from build123d import *

# Parameters (mm, degrees)
BOSS_EXTRUDE1_DEPTH = 3
SKETCH2_W           = 3
SKETCH2_H           = 3
CUT_EXTRUDE1_DEPTH  = 3
SKETCH3_R           = 1.5
CUT_EXTRUDE2_DEPTH  = 3
SKETCH4_W           = 3
SKETCH4_H           = 6
SKETCH4_H_2         = 3
CUT_EXTRUDE3_DEPTH  = 10


with BuildPart() as part:
    # Sketch1 → Boss-Extrude1 (new body)
    with BuildSketch(Plane(origin=(0, 0, 0), x_dir=(0, 0, -1), z_dir=(1, 0, 0))):
        Polygon((8, 30), (12.5, 30), (12.5, -30), (8, -30), (8, -27), (2, -27), (2, -30), (-2, -30), (-2, -27), (-8, -27), (-8, -30), (-12.5, -30), (-12.5, 30), (-8, 30), (-8, 27), (-2, 27), (-2, 30), (2, 30), (2, 27), (8, 27), align=None)
    extrude(amount=BOSS_EXTRUDE1_DEPTH)

    # Sketch2 → Cut-Extrude1 (cut)
    with BuildSketch(Plane(origin=(3, 0, 0), x_dir=(0, 0, -1), z_dir=(1, 0, 0))):
        with Locations((-5, 22.5)):
            Rectangle(SKETCH2_W, SKETCH2_H)
        with Locations((5, 22.5)):
            Rectangle(SKETCH2_W, SKETCH2_H)
        with Locations((5, -22.5)):
            Rectangle(SKETCH2_W, SKETCH2_H)
        with Locations((-5, -22.5)):
            Rectangle(SKETCH2_W, SKETCH2_H)
    extrude(amount=-CUT_EXTRUDE1_DEPTH, mode=Mode.SUBTRACT)

    # Sketch3 → Cut-Extrude2 (cut)
    with BuildSketch(Plane(origin=(3, 0, 0), x_dir=(0, 0, -1), z_dir=(1, 0, 0))):
        Circle(SKETCH3_R)
        with Locations((10, 0)):
            Circle(SKETCH3_R)
    extrude(amount=-CUT_EXTRUDE2_DEPTH, mode=Mode.SUBTRACT)

    # Sketch4 → Cut-Extrude3 (cut)
    with BuildSketch(Plane(origin=(3, 0, 0), x_dir=(0, 0, -1), z_dir=(1, 0, 0))):
        with Locations((-11, 0)):
            Rectangle(SKETCH4_W, SKETCH4_H)
        with Locations((-5, 5)):
            Rectangle(SKETCH4_W, SKETCH4_H_2)
        with Locations((-5, -5)):
            Rectangle(SKETCH4_W, SKETCH4_H_2)
    extrude(amount=-CUT_EXTRUDE3_DEPTH, mode=Mode.SUBTRACT)


solid = part.part
Could you check a few things on this model? Use its own coordinates, in mm. A direction names the side the tool comes from. Coordinates: 2 decimals unless noted, no trailing zeros. Loops run counter-clockwise (first coordinate to the right, second up) from the corner with the lowest first, then second, coordinate; pieces in that order, holes last.
1. For P1, Ø1.5, axis at x = 2, z = 4, coming from the -Y side; P2, Ø12, axis at y = 18.5, z = -3, coming from the -X side; P3, Ø1, axis at x = 2.5, y = -1.5, coming from the +Z side; P4, Ø1, axis at x = 1, z = -6.5, coming from the +Y side, each with a flat end and sliding along its axis, tell me the tip position at first contact or that it passes through.
2. Imagine slicing it at D-D (x = 0.65). Give the number of separate pieces and of enclosed holes in the cut face, and give its area (3 significant figures).
3. We'd pull the mould along Y, two halves only. Please class faces 1 (the face through (2, 24, -5)), 2 (the face through (1, 27, -5)), 3 (the face through (1, -27, 5)), 4 (the face through (2, 0, 9.5)): released by +Y, released by -Y, zero draft, split by the parting line, or undercut.
4. For faces 5 (the face through (1, -30, 10)), 6 (the face through (1, -29, -8)), 7 (the face through (2, 22, 3.5)), which set-ups out of +Z, -Z, +X, -X, +Y, -Y let a thin tool reach every point of the face, with its end or its side?
5. Imagine slicing it at B-B (y = 0). Please give me the cut outline in (x, z).
6. I need wall thicknesses on L1, parallel to Y at x = 1, z = -5; L2, parallel to Y at x = 0.5, z = 6; L3, parallel to Y at x = 1.6, z = 0. Which ranges of each line are inside material? Lowest first, please.
7. Imagine slicing it at C-C (z = -5). Please give me the cut outline in (x, y), and give its area (3 significant figures).
8. Imagine slicing it at A-A (z = -10). Please give me the cut outline in (x, y), and give its area (3 significant figures).
Computed values:
1. P1: stops at y = -27
1. P2: stops at x = 0
1. P3: stops at z = 9.5
1. P4: stops at y = 27
2. separate pieces: 1
2. enclosed holes: 8
2. area: 1,340 mm2
3. face 1: undercut
3. face 2: released by +Y
3. face 3: released by -Y
3. face 4: undercut
4. face 5: +Z, -Z, +X, -X, -Y
4. face 6: +X, -X, -Y
4. face 7: +X, -X
5. outline: (0, -12.5) - (3, -12.5) - (3, -11.5) - (0, -11.5) - close; (0, -8.5) - (3, -8.5) - (3, -1.5) - (0, -1.5) - close; (0, 1.5) - (3, 1.5) - (3, 9.5) - (0, 9.5) - close
6. L1: y = -27 to -24, -21 to 21, 24 to 27
6. L2: y = -27 to -24, -21 to -6.5, -3.5 to 3.5, 6.5 to 21, 24 to 27
6. L3: y = -30 to -1.5, 1.5 to 30
7. outline: (0, -27) - (3, -27) - (3, -24) - (0, -24) - close; (0, -21) - (3, -21) - (3, 21) - (0, 21) - close; (0, 24) - (3, 24) - (3, 27) - (0, 27) - close
7. area: 144 mm2
8. outline: (0, -30) - (3, -30) - (3, -1.5) - (0, -1.5) - close; (0, 1.5) - (3, 1.5) - (3, 30) - (0, 30) - close
8. area: 171 mm2
